For this review, take the finished solid that the model builds, in its own axes (mm). Coordinates: 2 decimals unless noted, no trailing zeros. Write each loop counter-clockwise with the first axis right and the second up, starting at its lowest first coordinate (ties: lowest second). Pieces come first, ordered by that corner, then holes. Notation, with made-up numbers: M -27,-39 L 5,-39 A17 ccw 5,-22 Z; hole C -15,84.5 d10. An arc over 180 degrees is marked long. One line per question, with ' | ' between items.
from build123d import *

# Parameters (mm, degrees)
F0_R     = 0.75
F1_DEPTH = 3


# Not quite as in the source:
# - a feature names something its author has since deleted; it is built from what else it names


with BuildPart() as f1:
    # F0 (on Top) → F1 (new body)
    with BuildSketch(Plane.XY):
        with BuildLine():
            ThreePointArc((-13.8337529302, 6.9912287808), (-6.1730560637, 14.2177135586), (4.3373536701, 14.8807715909))
            Line((4.3373536701, 14.8807715909), (-32.4411373594, 25.6007347374))
            ThreePointArc((-32.4411373594, 25.6007347374), (-35.456761187, 24.972624675), (-35.0323544011, 21.9216595489))
            Line((-35.0323544011, 21.9216595489), (-34.7850043318, 21.747447911))
            Line((-34.7850043318, 21.747447911), (-13.8337529302, 6.9912287808))
        make_face()
        with Locations((-33.6130708456, 23.6740913242)):
            Circle(F0_R, mode=Mode.SUBTRACT)
    extrude(amount=F1_DEPTH)


solid = f1.part
1) We need section C-C on x = -24. State the section outline as (y, z) points, then the cut area to 3 significant figures.
Responses:
outline: M 14.15,0 L 23.14,0 L 23.14,3 L 14.15,3 Z | area: 27.0 mm^2
2) To check wall thickness, follow line 1 along Y through (x, z) = (-32.5, 1.85); line 2 along Y through (x, z) = (-22, 1.6); line 3 along X through (y, z) = (14.25, 2.6). State the ranges of each line that lie inside material, in increasing order. Write a range as [from, to].
Responses:
line 1: [20.14, 25.64] | line 2: [12.74, 22.56] | line 3: [-24.14, -6.1]
3) We need section A-A on z = 1.45. State the section outline as (x, y) points (3 decimals).
Responses:
outline: M -35.032,21.922 L -13.834,6.991 A15.5 cw 4.337,14.881 L -32.441,25.601 A2.255 ccw Z; hole C -33.613,23.674 d1.5
4) We need section B-B on y = 12. State the section outline as (x, z) points, then the cut area to 3 significant figures.
Responses:
outline: M -20.95,0 L -9.81,0 L -9.81,3 L -20.95,3 Z | area: 33.4 mm^2
5) Insertion check: pin 1 Ø3 at (x, y) = (-10.5, 16) entering from -Z. The pin has a flat end and moves straight along its axis. Give the tip position at first contact, or say it passes through.
Responses:
pin 1: z = 0
6) The part is to be moulded in two halves that separate along Y. For faces 1 (the flat face through (-19, 17, 3)), 2 (the cylindrical face through (-33.2, 24.3, 1.5)), 3 (the cylindrical face through (-6.311, 14.157, 1.479)), 4 (the cylindrical face through (-35.43, 25.01, 1.48)), say which applies: +Y half, -Y half, draft (parallel to the pull), parting line (faces both ways), or undercut.
Responses:
face 1: draft | face 2: undercut | face 3: -Y half | face 4: parting line
